from build123d import *

# Parameters (mm, degrees)
SKETCH1_R           = 4.7
BOSS_EXTRUDE1_DEPTH = 5
SKETCH2_R           = 2.25
CUT_EXTRUDE1_DEPTH  = 9.317451533
CHAMFER1_SIZE       = 2.5


with BuildPart() as part:
    # Sketch1 → Boss-Extrude1 (new body)
    with BuildSketch(Plane(origin=(0, 0, 0), x_dir=(1, 0, 0), z_dir=(0, 1, 0))):
        with Locations(Location((0, 0, 0), (0, 0, 270))):
            Circle(SKETCH1_R)
    extrude(amount=BOSS_EXTRUDE1_DEPTH)

    # Sketch2 → Cut-Extrude1 (cut, through all)
    with BuildSketch(Plane(origin=(0, 5, 0), x_dir=(1, 0, 0), z_dir=(0, 1, 0))):
        with Locations(Location((0, 0, 0), (0, 0, 270))):
            Circle(SKETCH2_R)
    extrude(amount=-CUT_EXTRUDE1_DEPTH, mode=Mode.SUBTRACT)

    # Chamfer1
    # the kernel refuses this chamfer: 2.5 mm, written as the material it takes off along each edge
    with BuildSketch(Plane(origin=(0, 5, 0), x_dir=(0, 0, 1), z_dir=(-1, 0, 0))) as chamfer1_piece_1:
        Polygon((2.25 + CHAMFER1_SIZE, 0), (2.25, -CHAMFER1_SIZE), (2.25, 0), align=None)
    revolve(axis=Axis((0, 5, 0), (0, 1, 0)), mode=Mode.SUBTRACT)


solid = part.part
Here's how the part is built. I have some questions about the finished solid (model axes, mm). Coordinates: 2 decimals unless noted, no trailing zeros. Order: outer loops, then holes, each group sorted by start corner. A loop starts at its lowest first (then second) coordinate and runs counter-clockwise, first axis right, second up. Notation, with made-up numbers: M 44,73 L 77,73 A25 ccw 77,86 Z; hole C 65,53.25 d5. An arc over 180 degrees is marked long. Answer as CSV lines item,"result".
Item 1: Imagine slicing it at C-C on y = 1.75. Write out the boundary of the cut face in (x, z), plus the area to 3 significant figures.
Results found:
outline,"C 0,0 d9.4; hole C 0,0 d4.5"
area,"53.5 mm2"
Item 2: Imagine slicing it at B-B on z = 0. Write out the boundary of the cut face in (x, y).
Results found:
outline,"M -4.7,0 L -2.25,0 L -2.25,2.5 L -4.7,4.95 Z; M 2.25,0 L 4.7,0 L 4.7,4.95 L 2.25,2.5 Z"
Item 3: Imagine slicing it at D-D on y = 3. Write out the boundary of the cut face in (x, z), plus the area to 3 significant figures.
Results found:
outline,"C 0,0 d9.4; hole C 0,0 d5.5"
area,"45.6 mm2"
Item 4: If I drill on line 1 (X direction, y = 1.8, z = 0); line 2 (Z direction, x = 1.5, y = 2.4); line 3 (Z direction, x = -2, y = 4.75), over which ranges is the centre line in solid material (lowest first)?
Results found:
line 1,"-4.7 to -2.25, 2.25 to 4.7"
line 2,"-4.45 to -1.68, 1.68 to 4.45"
line 3,"-4.25 to -4.03, 4.03 to 4.25"
Item 5: Imagine slicing it at A-A on x = 0. Write out the boundary of the cut face in (y, z), plus the area to 3 significant figures.
Results found:
outline,"M 0,-4.7 L 4.95,-4.7 L 2.5,-2.25 L 0,-2.25 Z; M 0,2.25 L 2.5,2.25 L 4.95,4.7 L 0,4.7 Z"
area,"18.3 mm2"
Item 6: For pin 1 (1 mm diameter, centred on y = 0.5, z = -3.5, fed in from -X); pin 2 (2 mm diameter, centred on y = 0.5, z = 1.5, fed in from +X), each with a flat end and sliding along its axis, tell me the tip position at first contact or that it passes through.
Results found:
pin 1,"x = -3.62"
pin 2,"x = 4.67"
